Drawing for the job (mm, zero at the part's lowest x, y, z). Give positions to 0.01 mm unless a question says otherwise; leave off trailing zeros. Use a Markdown table: item, result. Add a question column.
(1) Flat gauge pins, fed straight in: pin 1 (1.5 mm diameter, centred on x = 3.18, z = 17.83, fed in from -Y); pin 2 (3 mm diameter, centred on x = 51.44, z = 17.83, fed in from +Y); pin 3 (1.5 mm diameter, centred on x = 7.5, y = 3, fed in from -Z); pin 4 (1 mm diameter, centred on y = 1, z = 11.5, fed in from +X) (1 decimal). Where does each tip first touch, or does it go through?
(2) Wall check: line 1 (X direction, y = 1.5, z = 3.95) (1 decimal); line 2 (Z direction, x = 48.26, y = 1.3) (1 decimal); line 3 (Z direction, x = 9.5, y = 0.35). Give the ranges that are in metal, low to high.
(3) Slice it at A-A (y = 4.2). Count the separate pieces of the cut face and the enclosed holes in it, then the cut area to 3 significant figures.
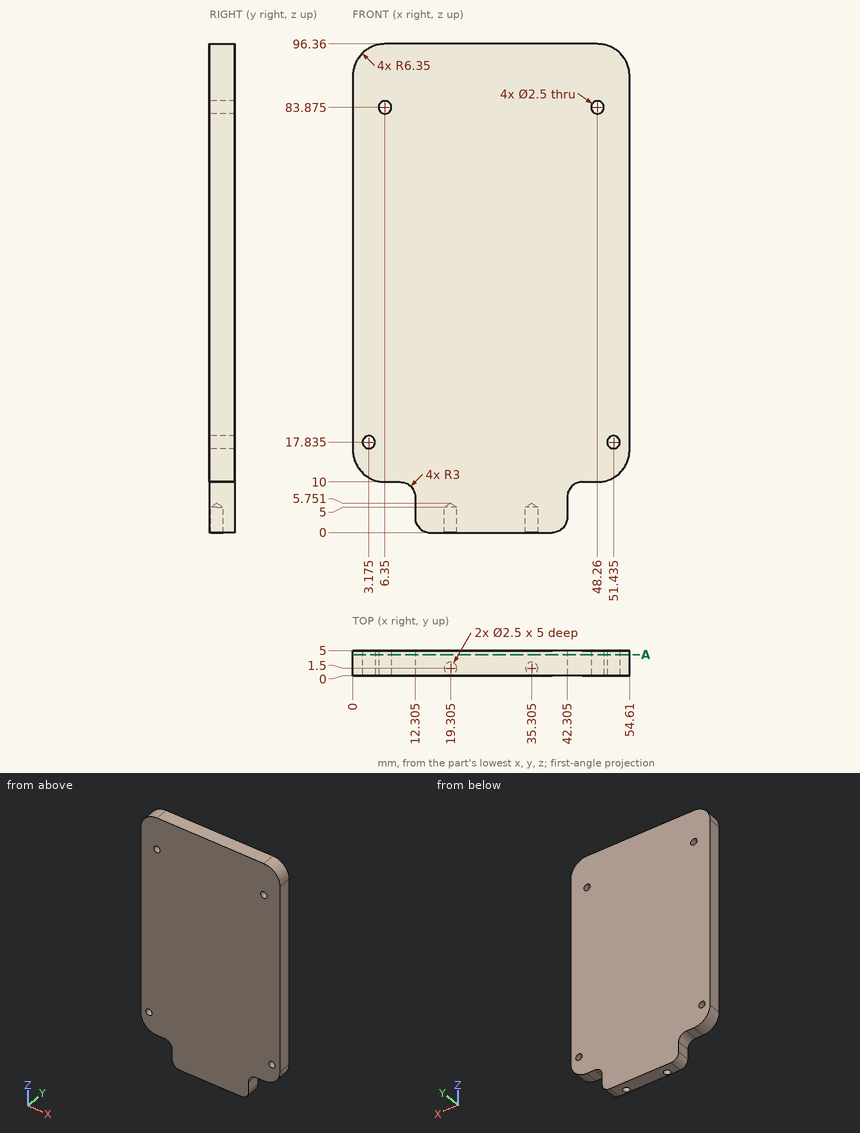
Solution:
| question | item | result |
|---|---|---|
| 1 | pin 1 | through |
| 1 | pin 2 | y = 5 |
| 1 | pin 3 | z = 10 |
| 1 | pin 4 | x = 52.9 |
| 2 | line 1 | 12.3 to 18.1, 20.6 to 34.1, 36.6 to 42.3 |
| 2 | line 2 | 10 to 82.6, 85.1 to 96.4 |
| 2 | line 3 | 9.99 to 96.36 |
| 3 | separate pieces | 1 |
| 3 | enclosed holes | 4 |
| 3 | area | 4,960 mm2 |
